Verification items for this drawing (mm, ordinates from the low corner). A direction names the side the tool comes from. Give positions to 0.01 mm unless a question says otherwise; leave off trailing zeros. Loops run counter-clockwise (first coordinate to the right, second up) from the corner with the lowest first, then second, coordinate; pieces in that order, holes last. Notation, with made-up numbers: M 85.25,65.25 L 99.25,65.25 A23 ccw 99.25,102.25 Z; hole C 0.25,-29.5 d2. An arc over 180 degrees is marked long. Answer in a Markdown table with one row per item.
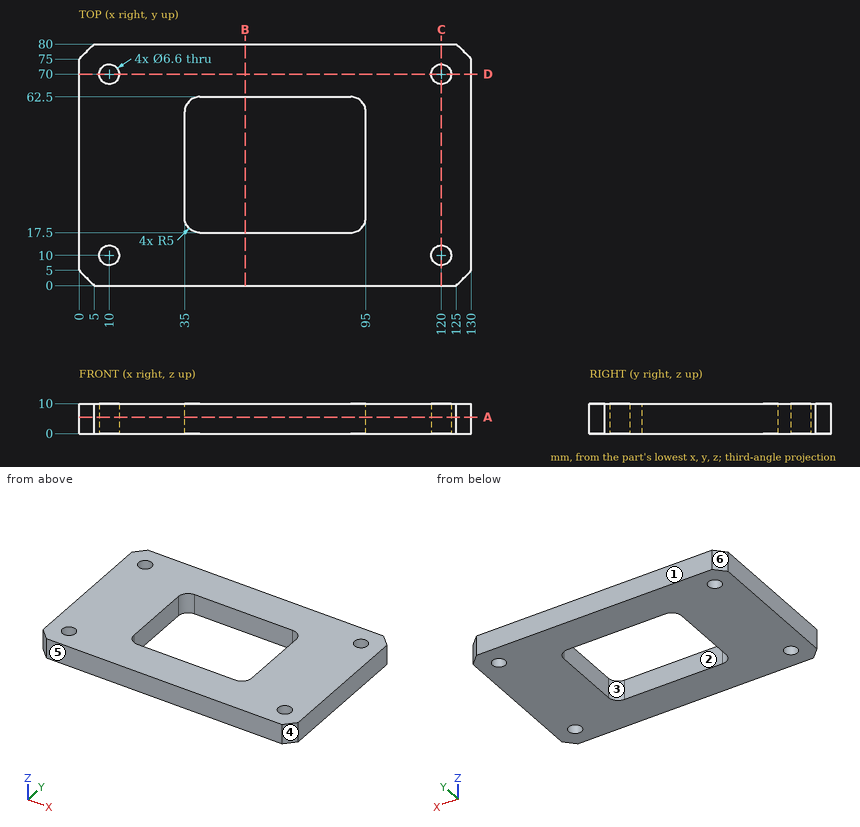
Item 1: Sectioned sample at A-A (z = 5.5). Record the cut outline in (x, y).
Reported:
| item | result |
|---|---|
| outline | M 0,5 L 5,0 L 125,0 L 130,5 L 130,75 L 125,80 L 5,80 L 0,75 Z; hole C 10,10 d6.6; hole C 10,70 d6.6; hole M 35,22.5 A5 ccw 40,17.5 L 90,17.5 A5 ccw 95,22.5 L 95,57.5 A5 ccw 90,62.5 L 40,62.5 A5 ccw 35,57.5 Z; hole C 120,10 d6.6; hole C 120,70 d6.6 |
Item 2: Sectioned sample at C-C (x = 120). Record the cut outline in (y, z).
Reported:
| item | result |
|---|---|
| outline | M 0,0 L 6.7,0 L 6.7,10 L 0,10 Z; M 13.3,0 L 66.7,0 L 66.7,10 L 13.3,10 Z; M 73.3,0 L 80,0 L 80,10 L 73.3,10 Z |
Item 3: Sectioned sample at B-B (x = 55). Record the cut outline in (y, z).
Reported:
| item | result |
|---|---|
| outline | M 0,0 L 17.5,0 L 17.5,10 L 0,10 Z; M 62.5,0 L 80,0 L 80,10 L 62.5,10 Z |
Item 4: Release check for a two-part mould opening along X. For the marked faces 3, 4, 5 and 6 record: released by +X, released by -X, zero draft, split by the parting line, or undercut.
Reported:
| item | result |
|---|---|
| face 3 | undercut |
| face 4 | released by +X |
| face 5 | zero draft |
| face 6 | released by -X |
Item 5: Sectioned sample at D-D (y = 70). Record the cut outline in (x, z), and give its area (3 significant figures).
Reported:
| item | result |
|---|---|
| outline | M 0,0 L 6.7,0 L 6.7,10 L 0,10 Z; M 13.3,0 L 116.7,0 L 116.7,10 L 13.3,10 Z; M 123.3,0 L 130,0 L 130,10 L 123.3,10 Z |
| area | 1,170 mm^2 |
Item 6: Scan lines: L1, parallel to Y at x = 120, z = 2.5; L2, parallel to X at y = 49, z = 8.5; L3, parallel to Y at x = 84.5, z = 3.25. Record each from-to range of solid material in increasing order. Write a range as [from, to].
Reported:
| item | result |
|---|---|
| L1 | y = [0, 6.7], [13.3, 66.7], [73.3, 80] |
| L2 | x = [0, 35], [95, 130] |
| L3 | y = [0, 17.5], [62.5, 80] |
Item 7: Tool access check on the marked faces 1 and 2. Record the directions out of +Z, -Z, +X, -X, +Y, -Y that give a thin tool (end or side, any length) a straight path to the whole face; none if there is none.
Reported:
| item | result |
|---|---|
| face 1 | +Z, -Z, +X, -X, +Y |
| face 2 | +Z, -Z |
Item 8: Go/stop test with a flat-tipped pin: pin 1 (5.5 mm diameter, centred on x = 10, y = 10, fed in from +Z). Record where the tip stops, or that it passes through.
Reported:
| item | result |
|---|---|
| pin 1 | passes through |
